Design review of the part built by this model. Coordinates are the model's own, in mm. A direction names the side the tool comes from. Round coordinates to 2 decimals unless told otherwise and drop trailing zeros. Order: outer loops, then holes, each group sorted by start corner. A loop starts at its lowest first (then second) coordinate and runs counter-clockwise, first axis right, second up.
Autodesk Inventor part; units mm, degrees
ref_plane "Start plane" through (0, 0, 0) normal (0, 0, 1) x (1, 0, 0)
ref_plane "End plane" through (0, 0, 994.771) normal (0, 0, 1) x (1, 0, 0)
ref_plane "Work Plane3" through (50.8, 38.1, 994.771) normal (-0.3827, 0, 0.9239) x (0.9239, 0, 0.3827)
ref_plane "Start plane" through (0, 0, 0) normal (0, 0, 1) x (1, 0, 0)
ref_plane "End plane" through (0, 0, 994.771) normal (0, 0, 1) x (1, 0, 0)
sketch "Sketch" plane through (0, 0, 0) normal (0, 0, 1) x (1, 0, 0)
  line L0 (0, 76.2) -> (0, 0)
  line L1 (0, 0) -> (50.8, 0)
  line L2 (50.8, 0) -> (50.8, 2.7625)
  line L3 (48.8, 4.7625) -> (12.6365, 4.7625)
  line L4 (4.7625, 12.6365) -> (4.7625, 74.2)
  line L5 (2.7625, 76.2) -> (0, 76.2)
  line L6 (-7.0414, 0) -> (21.5385, 0) construction
  line L7 (0, -8.0414) -> (0, 34.5385) construction
  arc A0 (4.7625, 12.6365) -> (12.6365, 4.7625) centre (12.6365, 12.6365) ccw
  arc A1 (50.8, 2.7625) -> (48.8, 4.7625) centre (48.8, 2.7625) ccw
  arc A2 (4.7625, 74.2) -> (2.7625, 76.2) centre (2.7625, 74.2) ccw
  line L8 (0, 93.5453) -> (0, -24.9725) construction
  line L9 (-18.6925, 0) -> (62.8653, 0) construction
  point P0 (50.8, 4.7625)
  point P1 (4.7625, 4.7625)
  point P2 (4.7625, 76.2)
  dimension "d12" = 4.7625
  dimension "d13" = 76.2
  dimension "d14" = 50.8
  dimension "d15" = 0
  dimension "d16" = 4.7625
  dimension "d17" = 0
  dimension "d18" = 7.874
  dimension "d19" = 2
extrude "Body" add sketch "Sketch" along normal up to surface (994.771 mm away) from surface at 0
sketch "Sketch3" plane through (0, 0, 0) normal (0, 0, 1) x (1, 0, 0)
  line L0 (0, 0) -> (10, 0)
ref_plane "Work Plane4" through (0, 0, 0) normal (0, -1, 0) x (1, 0, 0)
sketch "Sketch4" plane through (0, 0, 0) normal (0, -1, 0) x (1, 0, 0)
  line L0 (-2, 0) -> (12, 0)
  line L1 (-2, 994.771) -> (12, 994.771)
  dimension "d23" = 994.771
ref_plane "Work Plane3" through (50.8, 38.1, 994.771) normal (-0.3827, 0, 0.9239) x (0.9239, 0, 0.3827)
split "Split1" plane through (50.8, 38.1, 994.771) removes the side toward (-0.3827, 0, 0.9239)
equation "\"d12\" = G_T"
equation "\"d13\" = G_H"
equation "\"d14\" = G_W"
equation "\"d16\" = G_T"
equation "\"d18\" = G_IR"
equation "\"d4\" = G_L"
equation "\"G_W\" = 50.8"
equation "\"G_H\" = 76.2"
equation "\"G_T\" = 4.7625"
equation "\"G_ER\" = 4.064"
equation "\"G_IR\" = 7.874"
equation "\"G_L\" = d23"
equation "\"ex\" = 0"
equation "\"ey\" = 0"
equation "\"G_OFFSET_START\" = 0"
equation "\"G_OFFSET_END\" = 10.52102"
equation "\"d21\" = G_OFFSET_END + B_L"
equation "\"B_L\" = 984.25"
properties part number "ANSI L 3 x 2 x 3_16 00000001"
1) Take a section at B-B on y = 63. Give the boundary of the cut face in (x, z), plus the area to 3 significant figures.
Results:
outline: (0, 0) - (4.76, 0) - (4.76, 975.7) - (0, 973.73) - close
area: 4,640 mm2
2) For faces 1 (the face through (4.762, 43, 481)), 2 (the face through (25, 0, 490)), list the 3-axis set-ups (+Z, -Z, +X, -X, +Y, -Y) from which the entire face can be reached by the end or side of a thin tool; tool diameter is ignored.
Results:
face 1: +Z, -Z, +X, +Y
face 2: +Z, -Z, +X, -X, -Y
3) To check wall thickness, follow line 1 along X through (y, z) = (24.5, 772); line 2 along Y through (x, z) = (49.5, 491.5). State the ranges of each line that lie inside material, in increasing order.
Results:
line 1: x = 0 to 4.76
line 2: y = 0 to 4.64
4) Take a section at C-C on x = 41. Give the boundary of the cut face in (y, z), plus the area to 3 significant figures.
Results:
outline: (0, 0) - (4.76, 0) - (4.76, 990.71) - (0, 990.71) - close
area: 4,720 mm2
5) Take a section at A-A on z = 366. Give the boundary of the cut face in (x, y).
Results:
outline: (0, 0) - (50.8, 0) - (50.8, 2.76) arc R2 ccw to (48.8, 4.76) - (12.64, 4.76) arc R7.87 cw to (4.76, 12.64) - (4.76, 74.2) arc R2 ccw to (2.76, 76.2) - (0, 76.2) - close
6) Clearance check with flat-ended pins moving along their axes: P1, Ø2, axis at y = 59.5, z = 602, coming from the +X side; P2, Ø1, axis at y = 18.5, z = 138, coming from the -X side; P3, Ø3, axis at x = 6.5, y = 20.5, coming from the -Z side; P4, Ø1, axis at x = 44, z = 665, coming from the +Y side. State where each tip first meets the part, or that it passes through.
Results:
P1: stops at x = 4.76
P2: stops at x = 0
P3: passes through
P4: stops at y = 4.76
